For this review, take the finished solid that the model builds, in its own axes (mm). A direction names the side the tool comes from. Round coordinates to 2 decimals unless told otherwise and drop trailing zeros. Loops run counter-clockwise (first coordinate to the right, second up) from the corner with the lowest first, then second, coordinate; pieces in that order, holes last. Notation, with made-up numbers: (-12, -12.75) -> (9, -12.75) arc R14 ccw to (9, 14.25) -> close; hole circle Ø3 at (11, -35). An arc over 180 degrees is marked (long way). One line per question, with ' | ' between items. Start each with the question number.
1. For faces 1 (the face through (0, 15, 15)), 2 (the face through (20, 30, 20)), list the 3-axis set-ups (+Z, -Z, +X, -X, +Y, -Y) from which the entire face can be reached by the end or side of a thin tool; tool diameter is ignored.
2. Consider section C-C (y = 34). Write out the cut boundary in (x, z).
3. For pin 1 Ø1.5 at (x, z) = (25.5, 31.5) entering from +Y; pin 2 Ø2 at (y, z) = (29.5, 22.5) entering from -X; pin 3 Ø3 at (y, z) = (34, 27.5) entering from -X, all flat-tipped, find the tip position at first contact; note any pin that passes through.
4. Wall thickness on line 1 along Y through (x, z) = (29.5, 32.5); line 2 along X through (y, z) = (38.5, 20); line 3 along Z through (x, y) = (7.5, 28): over which ranges is each line inside the solid? List them lowest first.
5. Consider section B-B (x = 35). Write out the cut boundary in (y, z).
6. Consider section D-D (z = 31.5). Write out the cut boundary in (x, y), and give its area (3 significant figures).
7. Consider section A-A (z = 12). Write out the cut boundary in (x, y).
```python
from build123d import *

# Parameters (mm, degrees)
SKETCH1_W           = 40
SKETCH1_H           = 40
BOSS_EXTRUDE1_DEPTH = 40
SKETCH2_W           = 10
SKETCH2_H           = 20
CUT_EXTRUDE1_DEPTH  = 40
CUT_EXTRUDE2_DEPTH  = 20
SKETCH4_W           = 40
SKETCH4_H           = 20
BOSS_EXTRUDE2_DEPTH = 10


with BuildPart() as part:
    # Sketch1 → Boss-Extrude1 (new body)
    with BuildSketch(Plane.XY):
        with Locations((20, 20)):
            Rectangle(SKETCH1_W, SKETCH1_H)
    extrude(amount=BOSS_EXTRUDE1_DEPTH)

    # Sketch2 → Cut-Extrude1 (cut)
    with BuildSketch(Plane.ZY):
        with Locations((5, 30)):
            Rectangle(SKETCH2_W, SKETCH2_H)
    extrude(amount=-CUT_EXTRUDE1_DEPTH, mode=Mode.SUBTRACT)

    # Sketch3 → Cut-Extrude2 (cut)
    with BuildSketch(Plane(origin=(0, 40, 0), x_dir=(1, 0, 0), z_dir=(0, 1, 0))):
        Polygon((40, -30), (0, -10), (0, -40), (40, -40), align=None)
    extrude(amount=-CUT_EXTRUDE2_DEPTH, mode=Mode.SUBTRACT)

    # Sketch4 → Boss-Extrude2 (add)
    with BuildSketch(Plane(origin=(0, 0, 0), x_dir=(-1, 0, 0), z_dir=(0, 0, -1))):
        with Locations((-20, 30)):
            Rectangle(SKETCH4_W, SKETCH4_H)
    extrude(amount=-BOSS_EXTRUDE2_DEPTH)


solid = part.part
```
Answer block:
1) face 1: +Z, -Z, -X, +Y, -Y | face 2: +Z, -X, +Y
2) outline: (0, 0) -> (40, 0) -> (40, 30) -> (0, 10) -> close
3) pin 1: stops at y = 20 | pin 2: stops at x = 23 | pin 3: stops at x = 32
4) line 1: y = 0 to 20 | line 2: x = 20 to 40 | line 3: z = 0 to 13.75
5) outline: (0, 0) -> (40, 0) -> (40, 27.5) -> (20, 27.5) -> (20, 40) -> (0, 40) -> close
6) outline: (0, 0) -> (40, 0) -> (40, 20) -> (0, 20) -> close | area: 800 mm2
7) outline: (0, 0) -> (40, 0) -> (40, 40) -> (4, 40) -> (4, 20) -> (0, 20) -> close
